Verification items for the finished model (mm, model axes). Give positions to 0.01 mm unless a question says otherwise; leave off trailing zeros. Write each loop counter-clockwise with the first axis right and the second up, starting at its lowest first coordinate (ties: lowest second). Pieces come first, ordered by that corner, then holes. Notation, with made-up numbers: M 70,81.5 L 112,81.5 A23 ccw 112,115.5 Z; hole C 75.5,-11.5 d9. An arc over 180 degrees is marked long. Write item = value, one per line.
Autodesk Inventor part; units mm, degrees
ref_plane "YZ Plane" through (0, 0, 0) normal (1, 0, 0) x (0, 1, 0)
ref_plane "XZ Plane" through (0, 0, 0) normal (0, 1, 0) x (-1, 0, 0)
ref_plane "XY Plane" through (0, 0, 0) normal (0, 0, 1) x (1, 0, 0)
sketch "Náčrt1" plane through (0, 0, 0) normal (0, 1, 0) x (-1, 0, 0)
  line L0 (0, 0) -> (0, -15)
  line L1 (10, 0) -> (10, -15)
  line L2 (6, -5) -> (4, -5)
  line L3 (10, -15) -> (0, -15)
  line L4 (6, -5) -> (8, 0)
  line L5 (8, 0) -> (10, 0)
  line L6 (4, -5) -> (2, 0)
  line L7 (2, 0) -> (0, 0)
  dimension "d0" = 2
  dimension "d1" = 5
  dimension "d2" = 15
  dimension "d5" = 2
  dimension "d6" = 10
revolve "Rotace1" add sketch "Náčrt1" angle 360 about axis through (-10, 0, -15) along (1, 0, 0)
sketch "Náčrt2" plane through (0, 0, -15) normal (1, 0, 0) x (0, 0, -1)
  circle A0 centre (0, 0) radius 15
  circle A1 centre (0, 0) radius 10
  circle A2 centre (0, 0) radius 10.5
  point P0 (-15, 0)
  dimension "d8" = 21
extrude "Vysunutí1" cut sketch "Náčrt2" against normal blind 2.2 contours A1
sketch "Náčrt3" plane through (-10, 0, -15) normal (-1, 0, 0) x (0, 0, 1)
  circle A0 centre (0, 0) radius 15
  circle A1 centre (0, 0) radius 3
  point P0 (15, 0)
  dimension "d11" = 6
extrude "Vysunutí2" cut sketch "Náčrt3" against normal blind 1 contours A1
sketch "Náčrt4" plane through (-9, 0, -15) normal (-1, 0, 0) x (0, 0, 1)
  circle A0 centre (0, 0) radius 15
  circle A1 centre (0, 0) radius 10
  circle A2 centre (0, 0) radius 1.5
  point P0 (15, 0)
  dimension "d14" = 3
extrude "Vysunutí3" cut sketch "Náčrt4" against normal through all contours A2
sketch "Náčrt5" plane through (-10, 0, -15) normal (-1, 0, 0) x (0, 0, 1)
  circle A0 centre (0, 0) radius 3
  circle A1 centre (0, 0) radius 15
  circle A2 centre (0, 0) radius 1.5 construction
  circle A3 centre (0, 0) radius 7 construction
  circle A4 centre (7, 0) radius 1.4
  circle A5 centre (0, 0) radius 10 construction
  circle A6 centre (10, 0) radius 0.5
  circle A7 centre (0, 0) radius 15 construction
  line L0 (0, 15) -> (0, -15) construction
  circle A8 centre (-7, 0) radius 1.4
  point P0 (15, 0)
  dimension "d17" = 8
  dimension "d18" = 2.8
  dimension "d21" = 5
  dimension "d22" = 1
extrude "Vysunutí4" cut sketch "Náčrt5" against normal through all contours A4 | A6 | A8
sketch "Náčrt6" plane through (-10, 0, -15) normal (-1, 0, 0) x (0, 0, 1)
  circle A0 centre (7, 0) radius 1.4
  circle A1 centre (10, 0) radius 0.5
  circle A2 centre (0, 0) radius 3
  circle A3 centre (0, 0) radius 15
  point P0 (15, 0)
ref_plane "Pracovní rovina1" through (-6, 0, -15) normal (-1, 0, 0) x (0, 0, 1)
split "Rozdělit1" plane through (-6, 0, -15) removes the side toward (1, 0, 0)
sketch "Náčrt7" plane through (-10, 0, -15) normal (-1, 0, 0) x (0, 0, 1)
  circle A0 centre (7, 0) radius 1.4
  circle A1 centre (10, 0) radius 0.5
  circle A2 centre (-7, 0) radius 1.4
  circle A3 centre (0, 0) radius 3
  circle A4 centre (0, 0) radius 15
  circle A5 centre (-7, 0) radius 1.4
  circle A6 centre (-7, 0) radius 1.5
  circle A7 centre (7, 0) radius 1.5
  point P0 (15, 0)
  dimension "d24" = 3
  dimension "d25" = 3
extrude "Vysunutí5" cut sketch "Náčrt7" against normal through all contours A0 | A2 | A6
sketch "Sketch8" plane through (-6, 0, -15) normal (1, 0, 0) x (0, 0, -1)
  circle A0 centre (7, 0) radius 1.5
  circle A1 centre (-7, 0) radius 1.4
  arc A2 (-9.9875, -0.4998) -> (-9.9875, 0.4998) centre (-10, 0) ccw
  arc A3 (-9.9875, -0.4998) -> (-9.9875, 0.4998) centre (0, 0) ccw
  circle A4 centre (0, 0) radius 1.5
  circle A5 centre (-7, 0) radius 1.4
  circle A6 centre (7, 0) radius 1.5
  point P0 (-15, 0)
extrude "Extrusion6" add sketch "Sketch8" along normal blind 1.7 and the other way blind 4 contours A0 | A1
chamfer "Chamfer1" distance 0.5 angle 45 2 edges at (-4.3, 0, -6.6) (-4.3, 0, -20.5)
properties part number "bubinek_TOP"
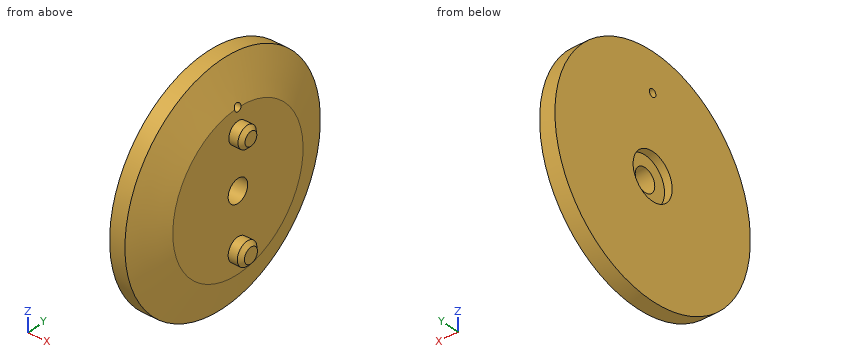
1) Cross-section at A-A on z = -15. Record the boundary of the cut face in (x, y), plus the area to 3 significant figures.
From the geometry:
outline = M -10,-15 L -8,-15 L -6,-10 L -6,-1.5 L -9,-1.5 L -9,-3 L -10,-3 Z; M -10,3 L -9,3 L -9,1.5 L -6,1.5 L -6,10 L -8,15 L -10,15 Z
area = 95.0 mm^2
2) Material ranges on probe 1 along X at (y, z) = (2.5, -20.5); probe 2 along Y at (x, z) = (-8.15, -5); probe 3 along X at (y, z) = (-3, -26), recorded low to high. Write a range as from..to.
From the geometry:
probe_1 = -10..-6
probe_2 = -11.18..-0.5, 0.5..11.18
probe_3 = -10..-6.56
3) Cross-section at C-C on x = -5.45. Record the boundary of the cut face in (y, z).
From the geometry:
outline = C 0,-22 d3; C 0,-8 d2.8
4) Cross-section at D-D on x = -9.55. Record the boundary of the cut face in (y, z), plus the area to 3 significant figures.
From the geometry:
outline = C 0,-15 d30; hole C 0,-15 d6; hole C 0,-5 d1
area = 678 mm^2
5) Cross-section at B-B on y = 0. Count the separate pieces of the cut face and the enclosed holes in it, plus the area to 3 significant figures.
From the geometry:
separate_pieces = 3
enclosed_holes = 0
area = 100 mm^2
6) Depth check by flat-ended pin: P1, Ø5, axis at y = 0, z = -15, coming from the -X side; P2, Ø6, axis at y = 4.5, z = -18, coming from the +X side. Enter the tip coordinate at first touch or a pass-through.
From the geometry:
P1 = -9
P2 = -6
